Geometry: final body of the model. Coordinates: model frame, mm. Face numbers are marked on the shaded views. A direction names the side the tool comes from. Give positions to 0.01 mm unless a question says otherwise; leave off trailing zeros. Loops run counter-clockwise (first coordinate to the right, second up) from the corner with the lowest first, then second, coordinate; pieces in that order, holes last.
from build123d import *

# Parameters (mm, degrees)
SKETCH1_R           = 16.5
BOSS_EXTRUDE1_DEPTH = 18
SKETCH2_R           = 3.5
BOSS_EXTRUDE2_DEPTH = 1.5
SKETCH3_R           = 1
BOSS_EXTRUDE3_DEPTH = 9
FILLET1_R           = 1
SKETCH4_R           = 1
CUT_EXTRUDE1_DEPTH  = 1.5
SKETCH5_R           = 3.5
BOSS_EXTRUDE4_DEPTH = 3
SKETCH6_R           = 15.8
SKETCH6_R_2         = 3.5
CUT_EXTRUDE2_DEPTH  = 0.5


with BuildPart() as part:
    # Sketch1 → Boss-Extrude1 (new body)
    with BuildSketch(Plane(origin=(0, 0, 0), x_dir=(1, 0, 0), z_dir=(0, 1, 0))):
        Circle(SKETCH1_R)
    extrude(amount=BOSS_EXTRUDE1_DEPTH)

    # Sketch2 → Boss-Extrude2 (add)
    with BuildSketch(Plane(origin=(0, 18, 0), x_dir=(1, 0, 0), z_dir=(0, 1, 0))):
        Circle(SKETCH2_R)
    extrude(amount=BOSS_EXTRUDE2_DEPTH)

    # Sketch3 → Boss-Extrude3 (add)
    with BuildSketch(Plane(origin=(0, 19.5, 0), x_dir=(1, 0, 0), z_dir=(0, 1, 0))):
        Circle(SKETCH3_R)
    extrude(amount=BOSS_EXTRUDE3_DEPTH)

    # Fillet1
    fillet1_edges = [part.edges().sort_by_distance(p)[0] for p in [
        (-16.5, 18, 0),
    ]]
    fillet(fillet1_edges, radius=FILLET1_R)

    # Sketch4 → Cut-Extrude1 (cut)
    with BuildSketch(Plane(origin=(0, 18, 0), x_dir=(1, 0, 0), z_dir=(0, 1, 0))):
        with Locations((11, 0)):
            Circle(SKETCH4_R)
        with Locations((-11, 0)):
            Circle(SKETCH4_R)
    extrude(amount=-CUT_EXTRUDE1_DEPTH, mode=Mode.SUBTRACT)

    # Sketch5 → Boss-Extrude4 (add)
    with BuildSketch(Plane.XZ):
        Circle(SKETCH5_R)
    extrude(amount=BOSS_EXTRUDE4_DEPTH)

    # Sketch6 → Cut-Extrude2 (cut)
    with BuildSketch(Plane.XZ):
        Circle(SKETCH6_R)
        Circle(SKETCH6_R_2, mode=Mode.SUBTRACT)
    extrude(amount=-CUT_EXTRUDE2_DEPTH, mode=Mode.SUBTRACT)


solid = part.part
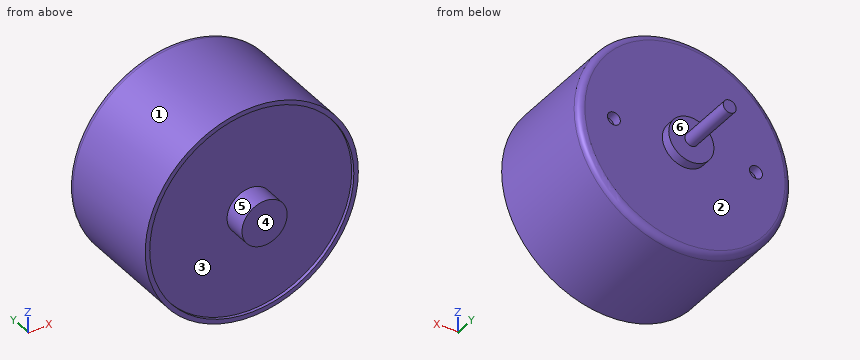
Item 1: Ray query, probe 1 along Z at (x, y) = (0, 0.2); probe 2 along X at (y, z) = (17, 0); probe 3 along Y at (x, z) = (4, 10). Return the intervals inside material, ascending.
Values follow:
probe 1: z = -16.5 to -15.8, -3.5 to 3.5, 15.8 to 16.5
probe 2: x = -16.5 to -12, -10 to 10, 12 to 16.5
probe 3: y = 0.5 to 18
Item 2: Pin query (flat end, axial travel): pin 1 (1.6 mm diameter, centred on x = -11, z = 0, fed in from +Y); pin 2 (12 mm diameter, centred on x = -10, z = 3.5, fed in from -Y); pin 3 (3 mm diameter, centred on x = 11, z = 0, fed in from +Y); pin 4 (2 mm diameter, centred on y = 24, z = 3.5, fed in from -X). Return the tip coordinate at first contact, or that it passes through.
Values follow:
pin 1: stops at y = 16.5
pin 2: stops at y = 0
pin 3: stops at y = 18
pin 4: passes through
Item 3: Draft query along Z for the marked faces 1, 2 and 3. Return one class per face: +Z half, -Z half, draft (parallel to the pull), parting line (faces both ways), or undercut.
Values follow:
face 1: parting line
face 2: draft
face 3: undercut
Item 4: Section query B-B on y = 8. Return loops of the section in (x, z), plus the area to 3 significant figures.
Values follow:
outline: circle Ø33 at (0, 0)
area: 855 mm2
Item 5: Set-up query: the marked faces 4, 5 and 6. Return all of +Z, -Z, +X, -X, +Y, -Y with unobstructed straight access to the full face (end or side cutting, diameter ignored); none if empty.
Values follow:
face 4: +Z, -Z, +X, -X, -Y
face 5: -Y
face 6: +Y
